from build123d import *

# Parameters (mm, degrees)
SKETCH1_R           = 1.6
SKETCH1_R_2         = 2.1
BOSS_EXTRUDE3_DEPTH = 2
BOSS_EXTRUDE4_DEPTH = 2
SKETCH4_W           = 66
SKETCH4_H           = 16.340111315
SKETCH4_H_2         = 24.741581589
CUT_EXTRUDE3_DEPTH  = 14.5
FILLET1_R           = 4
SKETCH5_W           = 26
SKETCH5_H           = 27
SKETCH5_R           = 6
BOSS_EXTRUDE5_DEPTH = 2
SKETCH6_W           = 5
SKETCH6_H           = 27
CUT_EXTRUDE4_DEPTH  = 14.5


with BuildPart() as part:
    # Sketch1 → Boss-Extrude3 (new body)
    with BuildSketch(Plane.XY):
        with BuildLine():
            Line((0, 3.5), (37.911912125, 3.5))
            Line((37.911912125, 3.5), (37.911912125, 13.97107578))
            Line((37.911912125, 13.97107578), (37.911912125, 40.97107578))
            Line((37.911912125, 40.97107578), (37.911912125, 51.44215156))
            Line((37.911912125, 51.44215156), (0, 51.44215156))
            ThreePointArc((0, 51.44215156), (-3.5, 54.94215156), (0, 58.44215156))
            Line((0, 58.44215156), (45.911912125, 58.44215156))
            Line((45.911912125, 58.44215156), (45.911912125, 51.44215156))
            Line((45.911912125, 51.44215156), (45.911912125, 48.97107578))
            Line((45.911912125, 48.97107578), (50.911912125, 48.97107578))
            Line((50.911912125, 48.97107578), (66.911912125, 48.97107578))
            Line((66.911912125, 48.97107578), (71.911912125, 48.97107578))
            Line((71.911912125, 48.97107578), (71.911912125, 51.44215156))
            Line((71.911912125, 51.44215156), (71.911912125, 58.44215156))
            Line((71.911912125, 58.44215156), (117.82382425, 58.44215156))
            ThreePointArc((117.82382425, 58.44215156), (121.32382425, 54.94215156), (117.82382425, 51.44215156))
            Line((117.82382425, 51.44215156), (79.911912125, 51.44215156))
            Line((79.911912125, 51.44215156), (79.911912125, 40.97107578))
            Line((79.911912125, 40.97107578), (79.911912125, 13.97107578))
            Line((79.911912125, 13.97107578), (79.911912125, 3.5))
            Line((79.911912125, 3.5), (117.82382425, 3.5))
            ThreePointArc((117.82382425, 3.5), (121.32382425, 0), (117.82382425, -3.5))
            Line((117.82382425, -3.5), (71.911912125, -3.5))
            Line((71.911912125, -3.5), (71.911912125, 3.5))
            Line((71.911912125, 3.5), (71.911912125, 5.97107578))
            Line((71.911912125, 5.97107578), (66.911912125, 5.97107578))
            Line((66.911912125, 5.97107578), (50.911912125, 5.97107578))
            Line((50.911912125, 5.97107578), (45.911912125, 5.97107578))
            Line((45.911912125, 5.97107578), (45.911912125, 3.5))
            Line((45.911912125, 3.5), (45.911912125, -3.5))
            Line((45.911912125, -3.5), (0, -3.5))
            ThreePointArc((0, -3.5), (-3.5, 0), (0, 3.5))
        make_face()
        with Locations((0, 54.94215156)):
            Circle(SKETCH1_R, mode=Mode.SUBTRACT)
        with Locations((117.82382425, 54.94215156)):
            Circle(SKETCH1_R, mode=Mode.SUBTRACT)
        with Locations((117.82382425, 0)):
            Circle(SKETCH1_R, mode=Mode.SUBTRACT)
        Circle(SKETCH1_R, mode=Mode.SUBTRACT)
        with Locations((66.911912125, 44.97107578)):
            Circle(SKETCH1_R_2, mode=Mode.SUBTRACT)
        with Locations((66.911912125, 9.97107578)):
            Circle(SKETCH1_R_2, mode=Mode.SUBTRACT)
        with Locations((50.911912125, 9.97107578)):
            Circle(SKETCH1_R_2, mode=Mode.SUBTRACT)
        with Locations((50.911912125, 44.97107578)):
            Circle(SKETCH1_R_2, mode=Mode.SUBTRACT)
        Polygon((66.911912125, 40.97107578), (50.911912125, 40.97107578), (45.911912125, 40.97107578), (45.911912125, 27.47107578), (45.911912125, 13.97107578), (50.911912125, 13.97107578), (66.911912125, 13.97107578), (71.911912125, 13.97107578), (71.911912125, 27.47107578), (71.911912125, 40.97107578), align=None, mode=Mode.SUBTRACT)
    extrude(amount=BOSS_EXTRUDE3_DEPTH)

    # Sketch3 → Boss-Extrude4 (add)
    with BuildSketch(Plane.XY.offset(2)):
        Polygon((71.911912125, 13.97107578), (99.911912125, 13.97107578), (99.911912125, 3.5), (91.911912125, 3.5), (91.911912125, 5.97107578), (71.911912125, 5.97107578), align=None)
        Polygon((91.911912125, 51.44215156), (99.911912125, 51.44215156), (99.911912125, 40.97107578), (71.911912125, 40.97107578), (71.911912125, 48.97107578), (91.911912125, 48.97107578), align=None)
        Polygon((45.911912125, 40.97107578), (17.911912125, 40.97107578), (17.911912125, 51.44215156), (25.911912125, 51.44215156), (25.911912125, 48.97107578), (45.911912125, 48.97107578), align=None)
        Polygon((25.911912125, 3.5), (17.911912125, 3.5), (17.911912125, 13.97107578), (45.911912125, 13.97107578), (45.911912125, 5.97107578), (25.911912125, 5.97107578), align=None)
    extrude(amount=-BOSS_EXTRUDE4_DEPTH)

    # Sketch4 → Cut-Extrude3 (cut)
    with BuildSketch(Plane.XY.offset(2)):
        with Locations((58.911912125, 57.141131438)):
            Rectangle(SKETCH4_W, SKETCH4_H)
        with Locations((58.911912125, -6.399715014)):
            Rectangle(SKETCH4_W, SKETCH4_H_2)
    extrude(amount=-CUT_EXTRUDE3_DEPTH, mode=Mode.SUBTRACT)

    # Fillet1
    fillet1_edges = [part.edges().sort_by_distance(p)[0] for p in [
        (99.911912125, 13.97107578, 1),
        (99.911912125, 3.5, 1),
        (91.911912125, 5.97107578, 1),
        (91.911912125, 48.97107578, 1),
        (99.911912125, 51.44215156, 1),
        (99.911912125, 40.97107578, 1),
        (17.911912125, 40.97107578, 1),
        (17.911912125, 51.44215156, 1),
        (25.911912125, 48.97107578, 1),
        (25.911912125, 5.97107578, 1),
        (17.911912125, 3.5, 1),
        (17.911912125, 13.97107578, 1),
        (91.911912125, 58.44215156, 1),
        (25.911912125, 58.44215156, 1),
        (91.911912125, -3.5, 1),
        (25.911912125, -3.5, 1),
    ]]
    fillet(fillet1_edges, radius=FILLET1_R)

    # Sketch5 → Boss-Extrude5 (add)
    with BuildSketch(Plane.XY.offset(2)):
        with Locations((58.911912125, 27.47107578)):
            Rectangle(SKETCH5_W, SKETCH5_H)
        with Locations((58.911912125, 27.47107578)):
            Circle(SKETCH5_R, mode=Mode.SUBTRACT)
    extrude(amount=-BOSS_EXTRUDE5_DEPTH)

    # Sketch6 → Cut-Extrude4 (cut)
    with BuildSketch(Plane.XY.offset(2)):
        with Locations((40.411912125, 27.47107578)):
            Rectangle(SKETCH6_W, SKETCH6_H)
        with Locations((77.411912125, 27.47107578)):
            Rectangle(SKETCH6_W, SKETCH6_H)
    extrude(amount=-CUT_EXTRUDE4_DEPTH, mode=Mode.SUBTRACT)


solid = part.part
Part model, mm, in its own coordinate system. A direction names the side the tool comes from. Give positions to 0.01 mm unless a question says otherwise; leave off trailing zeros. Write each loop counter-clockwise with the first axis right and the second up, starting at its lowest first coordinate (ties: lowest second). Pieces come first, ordered by that corner, then holes.
1) Cut at B-B on x = 78. Write the cut outline in (y, z), then the cut area to 3 significant figures.
Resolved:
outline: (5.97, 0) - (13.97, 0) - (13.97, 2) - (5.97, 2) - close; (40.97, 0) - (48.97, 0) - (48.97, 2) - (40.97, 2) - close
area: 32.0 mm2
2) Cut at A-A on x = 5. Write the cut outline in (y, z).
Resolved:
outline: (-3.5, 0) - (3.5, 0) - (3.5, 2) - (-3.5, 2) - close; (51.44, 0) - (58.44, 0) - (58.44, 2) - (51.44, 2) - close
3) Cut at C-C on y = 37. Write the cut outline in (x, z), then the cut area to 3 significant figures.
Resolved:
outline: (42.91, 0) - (74.91, 0) - (74.91, 2) - (42.91, 2) - close
area: 64.0 mm2
4) Pin check, flat tip, straight feed: pin 1 (0.7 mm diameter, centred on y = 1, z = 1.5, fed in from +X). Stop position of the tip, or through.
Resolved:
pin 1: stops at x = 121.26
5) Probe L1, parallel to Y at x = 51, z = 1.3; L2, parallel to X at y = 27.5, z = 1.5; L3, parallel to Y at x = 105, z = 1.5. List the from-to ranges inside material, lowest first.
Resolved:
L1: y = 5.97 to 7.87, 12.07 to 42.87, 47.07 to 48.97
L2: x = 42.91 to 52.91, 64.91 to 74.91
L3: y = -3.5 to 3.5, 51.44 to 58.44
6) Which spindle directions (+Z, -Z, +X, -X, +Y, -Y) get a long thin tool onto all of the face, cutting with end or side? Do faces 1 (the face through (90.77, 4.77, 0.99)), 2 (the face through (93.115, 57.302, 0.986)), 3 (the face through (98.77, 12.77, 0.99)). Say none if no direction does.
Resolved:
face 1: +Z, -Z, -Y
face 2: +Z, -Z, +Y
face 3: +Z, -Z, +X
7) Two-plate mould, pull along X, no slides. Class faces 4 (the face through (58, 35, 2)), 5 (the face through (98.71, 42.11, 0.99)), 6 (the face through (64.814, 10.063, 0.986)): released by +X, released by -X, zero draft, split by the parting line, or undercut.
Resolved:
face 4: zero draft
face 5: released by +X
face 6: undercut
8) Cut at D-D on z = 1.25. State how many separate pieces and enclosed holes the cut face has, then the cut area to 3 significant figures.
Resolved:
separate pieces: 1
enclosed holes: 9
area: 2,860 mm2
